Geometry: see drawing. Coordinates: mm, zero at the bounding-box minimum. Give positions to 0.01 mm unless a question says otherwise; leave off trailing zeros. Order: outer loops, then holes, each group sorted by start corner. A loop starts at its lowest first (then second) coordinate and runs counter-clockwise, first axis right, second up. Notation, with made-up numbers: M 46.25,74 L 50.25,74 A17 cw 50.25,85 Z; hole C -39.75,63 d2. An arc over 180 degrees is marked long. Return JSON: item names as keys, results as strings.
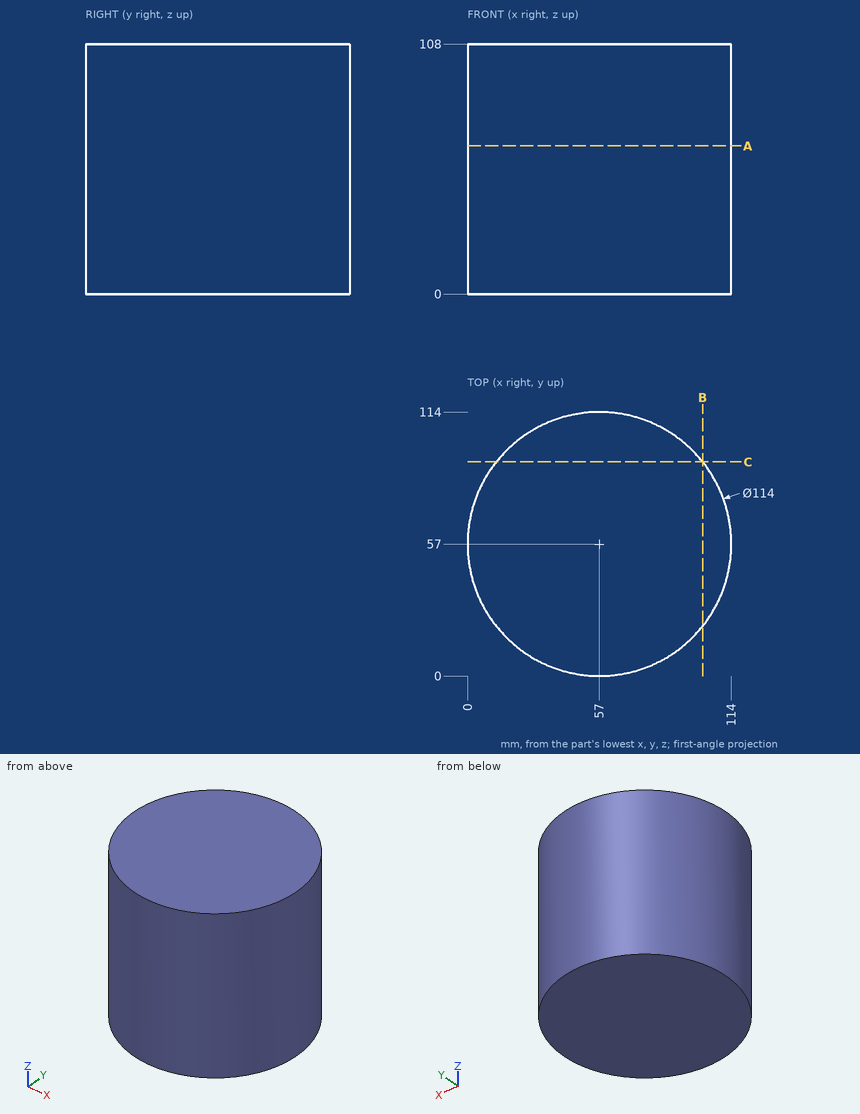
1. First-contact query: pin 1 (12 mm diameter, centred on x = 42, z = 19.5, fed in from -Y) (3 decimals); pin 2 (10 mm diameter, centred on y = 90.5, z = 49, fed in from +X); pin 3 (3 mm diameter, centred on y = 79.5, z = 16, fed in from -X). Flat tips, straight axial feed; report the tip coordinate or a pass-through.
Evaluation:
{"pin 1": "stops at y = 0.715", "pin 2": "stops at x = 106.36", "pin 3": "stops at x = 4.01"}
2. Section query C-C (y = 92.5). Return loops of the section in (x, z).
Evaluation:
{"outline": "M 12.4,0 L 101.6,0 L 101.6,108 L 12.4,108 Z"}
3. Section query B-B (x = 101.5). Return loops of the section in (y, z), then the cut area to 3 significant figures.
Evaluation:
{"outline": "M 21.38,0 L 92.62,0 L 92.62,108 L 21.38,108 Z", "area": "7,690 mm^2"}
4. Ray query, probe 1 along X at (y, z) = (82.5, 86); probe 2 along Y at (x, z) = (93.5, 22); probe 3 along Y at (x, z) = (6, 12). Return the intervals inside material, ascending.
Evaluation:
{"probe 1": "x = 6.02 to 107.98", "probe 2": "y = 13.22 to 100.78", "probe 3": "y = 31.54 to 82.46"}
5. Section query A-A (z = 64). Return loops of the section in (x, y).
Evaluation:
{"outline": "C 57,57 d114"}
